```python
from build123d import *

# Parameters (mm, degrees)
F1_DEPTH = 10
F4_DEPTH = 10.001
F6_D     = 3.556
F7_R     = 5


# Not quite as in the source:
# - a feature of the source that left no trace in its solid (it failed there, or was rolled back) is left out
# - a feature names something its author has since deleted; it is built from what else it names


with BuildPart() as f1:
    # F0 (on Top) → F1 (new body)
    with BuildSketch(Plane.XY):
        with BuildLine():
            ThreePointArc((16.1705551086, 23.468343518), (24.7491207645, 14.1326225939), (28.4297379517, 2))
            Line((28.4297379517, 2), (28.4297379517, 7))
            Line((28.4297379517, 7), (32.7604945018, 7))
            ThreePointArc((32.7604945018, 7), (26.8945535829, 19.9733068763), (16.1705551086, 29.3387652685))
            Line((16.1705551086, 29.3387652685), (16.1705551086, 23.468343518))
        make_face()
        with BuildLine():
            ThreePointArc((-16.1705551086, 23.468343518), (0, 28.5), (16.1705551086, 23.468343518))
            Line((16.1705551086, 23.468343518), (16.1705551086, 29.3387652685))
            Line((16.1705551086, 29.3387652685), (-16.1705551086, 29.3387652685))
            Line((-16.1705551086, 29.3387652685), (-16.1705551086, 23.468343518))
        make_face()
        with BuildLine():
            ThreePointArc((-28.4297379517, 2), (-24.7491207645, 14.1326225939), (-16.1705551086, 23.468343518))
            Line((-16.1705551086, 23.468343518), (-16.1705551086, 29.3387652685))
            ThreePointArc((-16.1705551086, 29.3387652685), (-26.8945535829, 19.9733068763), (-32.7604945018, 7))
            Line((-32.7604945018, 7), (-28.4297379517, 7))
            Line((-28.4297379517, 7), (-28.4297379517, 2))
        make_face()
        with BuildLine():
            Line((-48.4297379517, 2), (-33.4402452144, 2))
            ThreePointArc((-33.4402452144, 2), (-33.1946454228, 4.5128167765), (-32.7604945018, 7))
            Line((-32.7604945018, 7), (-48.4297379517, 7))
            Line((-48.4297379517, 7), (-48.4297379517, 2))
        make_face()
        with BuildLine():
            Line((-33.4402452144, 2), (-28.4297379517, 2))
            Line((-28.4297379517, 2), (-28.4297379517, 7))
            Line((-28.4297379517, 7), (-32.7604945018, 7))
            ThreePointArc((-32.7604945018, 7), (-33.1946454228, 4.5128167765), (-33.4402452144, 2))
        make_face()
        with BuildLine():
            Line((28.4297379517, 7), (28.4297379517, 2))
            Line((28.4297379517, 2), (33.4402452144, 2))
            ThreePointArc((33.4402452144, 2), (33.1946454228, 4.5128167765), (32.7604945018, 7))
            Line((32.7604945018, 7), (28.4297379517, 7))
        make_face()
        with BuildLine():
            ThreePointArc((32.7604945018, 7), (33.1946454228, 4.5128167765), (33.4402452144, 2))
            Line((33.4402452144, 2), (48.4297379517, 2))
            Line((48.4297379517, 2), (48.4297379517, 7))
            Line((48.4297379517, 7), (32.7604945018, 7))
        make_face()
        with BuildLine():
            Line((-16.1705551086, 29.3387652685), (16.1705551086, 29.3387652685))
            ThreePointArc((16.1705551086, 29.3387652685), (8.3486935036, 32.4430164563), (1.811e-07, 33.5))
            ThreePointArc((1.811e-07, 33.5), (-8.3486933282, 32.4430165014), (-16.1705551086, 29.3387652685))
        make_face()
    extrude(amount=F1_DEPTH)

    # F0 (on Top) → F4 (cut, through all)
    with BuildSketch(Plane.XY):
        with BuildLine():
            Line((-16.1705551086, 23.468343518), (16.1705551086, 23.468343518))
            ThreePointArc((16.1705551086, 23.468343518), (0, 28.5), (-16.1705551086, 23.468343518))
        make_face()
    extrude(amount=F4_DEPTH, mode=Mode.SUBTRACT)

    # F6 (through all)
    with Locations(Plane.XZ.offset(-2)):
        with Locations((-39.116, 4.78035165), (39.116, 4.78035165)):
            Hole(F6_D / 2)

    # F7
    f7_edges = [f1.edges().sort_by_distance(p)[0] for p in [
        (-32.760495, 7, 5),
        (32.760495, 7, 5),
    ]]
    fillet(f7_edges, radius=F7_R)


solid = f1.part
```
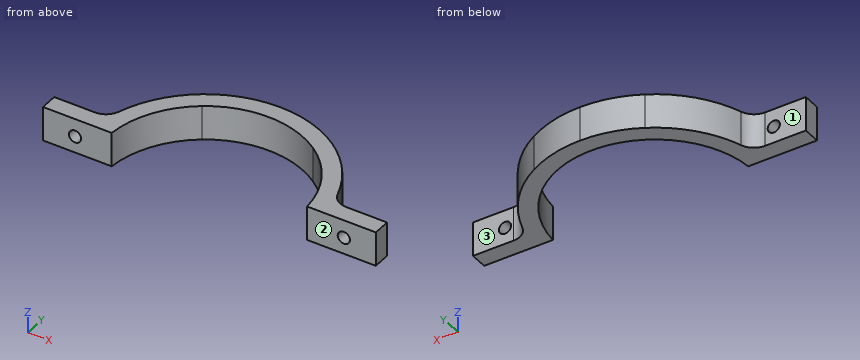
The listing builds one solid part. Answer for the finished solid, in the listing's coordinates (mm). Face numbers are marked on the shaded views. A direction names the side the tool comes from. Give positions to 0.01 mm unless a question says otherwise; leave off trailing zeros. Write each loop counter-clockwise with the first axis right and the second up, starting at its lowest first coordinate (ties: lowest second). Pieces come first, ordered by that corner, then holes. Notation, with made-up numbers: (-19, 12.25) - (2, 12.25) arc R37 cw to (2, 49.25) - close; hole circle Ø2 at (61.25, -28.5). An arc over 180 degrees is marked (long way). Use one line per item in the form item = value. Start each with the question number.
1) Flat-ended cylindrical pins translate along their axes: pin 1 Ø3 at (x, z) = (-41.5, 6) entering from +Y; pin 2 Ø1 at (x, y) = (24.5, 23.5) entering from +Z; pin 3 Ø6 at (y, z) = (15, 2.5) entering from +X. Find the tip coordinate at first contact, or state that the pin passes through.
2) A tool of negligible diameter and unlimited length cuts with its end or side. For the marked faces 1, 2 and 3, from which of +Z, -Z, +X, -X, +Y, -Y can it reach the whole face along a straight path? Write none if from no direction.
3) Find section D-D on x = -4.5. Determine the outline of the cut face in (y, z).
4) Consider line 1 along X through (y, z) = (22, 8.25); line 2 along Y through (x, z) = (-36.5, 6.75); line 3 along X through (y, z) = (15, 5). Determine where each line is inside the solid, lowest interval first. Write a range as from..to.
5) Find section A-A on y = 19. Determine the outline of the cut face in (x, z).
6) Find section B-B on y = 4.5. Determine the outline of the cut face in (x, z).
7) Find section C-C on y = 9. Determine the outline of the cut face in (x, z).
Geometry results:
q1.pin_1 = 7
q1.pin_2 = 10
q1.pin_3 = 31.28
q2.face_1 = +Z, -Z, -X, +Y
q2.face_2 = +Z, -Z, +X, -X, -Y
q2.face_3 = +Z, -Z, +X, +Y
q3.outline = (28.14, 0) - (33.2, 0) - (33.2, 10) - (28.14, 10) - close
q4.line_1 = -25.26..-18.12, 18.12..25.26
q4.line_2 = 2..7
q4.line_3 = -29.95..-24.23, 24.23..29.95
q5.outline = (-27.59, 0) - (-21.24, 0) - (-21.24, 10) - (-27.59, 10) - close; (21.24, 0) - (27.59, 0) - (27.59, 10) - (21.24, 10) - close
q6.outline = (-48.43, 0) - (-28.14, 0) - (-28.14, 10) - (-48.43, 10) - close; (28.14, 0) - (48.43, 0) - (48.43, 10) - (28.14, 10) - close; hole circle Ø3.56 at (-39.12, 4.78); hole circle Ø3.56 at (39.12, 4.78)
q7.outline = (-32.58, 0) - (-27.04, 0) - (-27.04, 10) - (-32.58, 10) - close; (27.04, 0) - (32.58, 0) - (32.58, 10) - (27.04, 10) - close
